```python
from build123d import *

# Parameters (mm, degrees)
SKETCH1_W           = 75
SKETCH1_H           = 35
BOSS_EXTRUDE1_DEPTH = 30
SKETCH2_W           = 20
SKETCH2_H           = 30
CUT_EXTRUDE1_DEPTH  = 25
SKETCH3_W           = 35
SKETCH3_H           = 20
CUT_EXTRUDE2_DEPTH  = 36
SKETCH4_R           = 7.5
CUT_EXTRUDE3_DEPTH  = 11
SKETCH5_R           = 5
CUT_EXTRUDE4_DEPTH  = 76


with BuildPart() as part:
    # Sketch1 → Boss-Extrude1 (new body)
    with BuildSketch(Plane(origin=(0, 0, 0), x_dir=(1, 0, 0), z_dir=(0, 1, 0))):
        with Locations((37.5, 17.5)):
            Rectangle(SKETCH1_W, SKETCH1_H)
    extrude(amount=BOSS_EXTRUDE1_DEPTH)

    # Sketch2 → Cut-Extrude1 (cut)
    with BuildSketch(Plane.XY):
        with Locations((20, 15)):
            Rectangle(SKETCH2_W, SKETCH2_H)
    extrude(amount=-CUT_EXTRUDE1_DEPTH, mode=Mode.SUBTRACT)

    # Sketch3 → Cut-Extrude2 (cut, through all)
    with BuildSketch(Plane.XY):
        with Locations((57.5, 20)):
            Rectangle(SKETCH3_W, SKETCH3_H)
    extrude(amount=-CUT_EXTRUDE2_DEPTH, mode=Mode.SUBTRACT)

    # Sketch4 → Cut-Extrude3 (cut, through all)
    with BuildSketch(Plane(origin=(0, 10, 0), x_dir=(1, 0, 0), z_dir=(0, 1, 0))):
        with Locations((57.5, 17.5)):
            Circle(SKETCH4_R)
    extrude(amount=-CUT_EXTRUDE3_DEPTH, mode=Mode.SUBTRACT)

    # Sketch5 → Cut-Extrude4 (cut, through all)
    with BuildSketch(Plane.ZY):
        with Locations((-10, 20)):
            Circle(SKETCH5_R)
    extrude(amount=-CUT_EXTRUDE4_DEPTH, mode=Mode.SUBTRACT)


solid = part.part
```
For this review, take the finished solid that the model builds, in its own axes (mm). A direction names the side the tool comes from. Coordinates: 2 decimals unless noted, no trailing zeros. Write each loop counter-clockwise with the first axis right and the second up, starting at its lowest first coordinate (ties: lowest second). Pieces come first, ordered by that corner, then holes. Notation, with made-up numbers: (24.5, 64) -> (74.5, 64) arc R31 cw to (74.5, 99) -> close; hole circle Ø10 at (88.5, -1.75). An arc over 180 degrees is marked (long way). Put each result on its own line as item: value.
Q1. Clearance check with flat-ended pins moving along their axes: pin 1 Ø13 at (y, z) = (20, -10) entering from +X; pin 2 Ø8 at (y, z) = (20, -10) entering from +X. State where each tip first meets the part, or that it passes through.
From the geometry:
pin 1: stops at x = 40
pin 2: passes through
Q2. Take a section at B-B, the plane y = 24. State the section outline as (x, z) points, then the cut area to 3 significant figures.
From the geometry:
outline: (0, -35) -> (40, -35) -> (40, -13) -> (30, -13) -> (30, -25) -> (10, -25) -> (10, -13) -> (0, -13) -> close; (0, -7) -> (10, -7) -> (10, 0) -> (0, 0) -> close; (30, -7) -> (40, -7) -> (40, 0) -> (30, 0) -> close
area: 780 mm2
Q3. Take a section at C-C, the plane z = -17.5. State the section outline as (x, y) points, then the cut area to 3 significant figures.
From the geometry:
outline: (0, 0) -> (10, 0) -> (10, 30) -> (0, 30) -> close; (30, 0) -> (50, 0) -> (50, 10) -> (40, 10) -> (40, 30) -> (30, 30) -> close; (65, 0) -> (75, 0) -> (75, 10) -> (65, 10) -> close
area: 800 mm2
Q4. Take a section at D-D, the plane x = 5. State the section outline as (y, z) points, then the cut area to 3 significant figures.
From the geometry:
outline: (0, -35) -> (30, -35) -> (30, 0) -> (0, 0) -> close; hole circle Ø10 at (20, -10)
area: 971 mm2
Q5. Tool access review of faces 5 (the flat face through (5, 15, 0)), 6 (the flat face through (30, 15, -12)), 7 (the flat face through (40, 20, -17)): name each direction out of +Z, -Z, +X, -X, +Y, -Y from which nothing blocks a thin tool from reaching the whole face with its end or side.
From the geometry:
face 5: +Z, +X, -X, +Y, -Y
face 6: +Z, +Y, -Y
face 7: +Z, -Z, +X, +Y
Q6. The part is to be moulded in two halves that separate along Z. For faces 1 (the flat face through (20, 30, -26)), 2 (the cylindrical face through (4.93, 15.564, -7.693)), 3 (the flat face through (20, 15, -25)), 4 (the cylindrical face through (34.93, 15.564, -7.693)), say which applies: +Z half, -Z half, draft (parallel to the pull), parting line (faces both ways), or undercut.
From the geometry:
face 1: draft
face 2: undercut
face 3: +Z half
face 4: undercut
Q7. Wall thickness on L1, parallel to X at y = 10.75, z = -5; L2, parallel to X at y = 7.25, z = -11.5; L3, parallel to Z at x = 57.5, y = 6.75: over which ranges is each line inside the solid? List them lowest first.
From the geometry:
L1: x = 0 to 10, 30 to 40
L2: x = 0 to 10, 30 to 53, 62 to 75
L3: z = -35 to -25, -10 to 0
Q8. Take a section at A-A, the plane x = 57.5. State the section outline as (y, z) points, then the cut area to 3 significant figures.
From the geometry:
outline: (0, -35) -> (10, -35) -> (10, -25) -> (0, -25) -> close; (0, -10) -> (10, -10) -> (10, 0) -> (0, 0) -> close
area: 200 mm2
